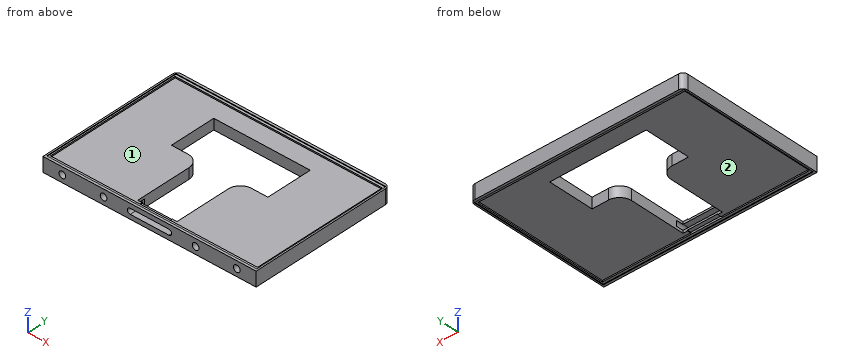
from build123d import *

# Parameters (mm, degrees)
SKETCH_1_W           = 176
SKETCH_1_H           = 120
EXTRUDE_1_DEPTH      = 12
SKETCH_2_W           = 171
SKETCH_2_H           = 112
CUT_EXTRUDE_1_DEPTH  = 1.6
SKETCH_3_W           = 171
SKETCH_3_H           = 112
CUT_EXTRUDE_2_DEPTH  = 1.6
SKETCH_5_W           = 173.4
SKETCH_5_H           = 116
CUT_EXTRUDE_3_DEPTH  = 0.5
SKETCH_6_W           = 173.4
SKETCH_6_H           = 116
CUT_EXTRUDE_4_DEPTH  = 0.5
SKETCH_7_W           = 32.5
SKETCH_7_H           = 56
CUT_EXTRUDE_5_DEPTH  = 108.014765336
SKETCH_8_W           = 25
SKETCH_8_H           = 5
CUT_EXTRUDE_6_DEPTH  = 0.5
SKETCH_9_W           = 25
SKETCH_9_H           = 5
CUT_EXTRUDE_7_DEPTH  = 0.5
FILLET_1_R           = 4
FILLET_2_R           = 4
SKETCH_28_R          = 2.75
CUT_EXTRUDE_16_DEPTH = 5.5
CUT_EXTRUDE_17_DEPTH = 13
SKETCH_31_W          = 79.660251382
SKETCH_31_H          = 38
CUT_EXTRUDE_18_DEPTH = 108.014765336
FILLET_3_R           = 10
FILLET_4_R           = 10


with BuildPart() as part:
    # 草图1 → 凸台-拉伸1 (new body)
    with BuildSketch(Plane.XY):
        Rectangle(SKETCH_1_W, SKETCH_1_H)
    extrude(amount=EXTRUDE_1_DEPTH)

    # 草图2 → 切除-拉伸1 (cut)
    with BuildSketch(Plane.XY.offset(12)):
        Rectangle(SKETCH_2_W, SKETCH_2_H)
    extrude(amount=-CUT_EXTRUDE_1_DEPTH, mode=Mode.SUBTRACT)

    # 草图3 → 切除-拉伸2 (cut)
    with BuildSketch(Plane(origin=(0, 0, 0), x_dir=(-1, 0, 0), z_dir=(0, 0, -1))):
        Rectangle(SKETCH_3_W, SKETCH_3_H)
    extrude(amount=-CUT_EXTRUDE_2_DEPTH, mode=Mode.SUBTRACT)

    # 草图5 → 切除-拉伸3 (cut)
    with BuildSketch(Plane(origin=(0, 0, 0), x_dir=(-1, 0, 0), z_dir=(0, 0, -1))):
        Rectangle(SKETCH_5_W, SKETCH_5_H)
    extrude(amount=-CUT_EXTRUDE_3_DEPTH, mode=Mode.SUBTRACT)

    # 草图6 → 切除-拉伸4 (cut)
    with BuildSketch(Plane.XY.offset(12)):
        Rectangle(SKETCH_6_W, SKETCH_6_H)
    extrude(amount=-CUT_EXTRUDE_4_DEPTH, mode=Mode.SUBTRACT)

    # 草图7 → 切除-拉伸5 (cut, through all)
    with BuildSketch(Plane(origin=(0, 0, 1.6), x_dir=(-1, 0, 0), z_dir=(0, 0, -1))):
        with Locations((0, -25)):
            Rectangle(SKETCH_7_W, SKETCH_7_H)
    extrude(amount=-CUT_EXTRUDE_5_DEPTH, mode=Mode.SUBTRACT)

    # 草图8 → 切除-拉伸6 (cut)
    with BuildSketch(Plane(origin=(0, 0, 1.6), x_dir=(-1, 0, 0), z_dir=(0, 0, -1))):
        with Locations((0, -53.5)):
            Rectangle(SKETCH_8_W, SKETCH_8_H)
    extrude(amount=-CUT_EXTRUDE_6_DEPTH, mode=Mode.SUBTRACT)

    # 草图9 → 切除-拉伸7 (cut)
    with BuildSketch(Plane.XY.offset(10.4)):
        with Locations((0, -53.5)):
            Rectangle(SKETCH_9_W, SKETCH_9_H)
    extrude(amount=-CUT_EXTRUDE_7_DEPTH, mode=Mode.SUBTRACT)

    # 圆角1
    fillet_1_edges = [part.edges().sort_by_distance(p)[0] for p in [
        (-88, 60, 6),
    ]]
    fillet(fillet_1_edges, radius=FILLET_1_R)

    # 圆角2
    fillet_2_edges = [part.edges().sort_by_distance(p)[0] for p in [
        (88, 60, 6),
    ]]
    fillet(fillet_2_edges, radius=FILLET_2_R)

    # 草图28 → 切除-拉伸16 (cut)
    with BuildSketch(Plane(origin=(0, -60, 0), x_dir=(-1, 0, 0), z_dir=(0, -1, 0))):
        with Locations(Location((-72, -6, 0), (0, 0, 180))):
            Circle(SKETCH_28_R)
        with Locations(Location((-38, -6, 0), (0, 0, 180))):
            Circle(SKETCH_28_R)
        with Locations(Location((38, -6, 0), (0, 0, 180))):
            Circle(SKETCH_28_R)
        with Locations(Location((72, -6, 0), (0, 0, 180))):
            Circle(SKETCH_28_R)
    extrude(amount=-CUT_EXTRUDE_16_DEPTH, mode=Mode.SUBTRACT)

    # 草图29 → 切除-拉伸17 (cut)
    with BuildSketch(Plane.XZ.offset(60)):
        with BuildLine():
            Line((-16, 8.25), (16, 8.25))
            ThreePointArc((16, 8.25), (18.25, 6), (16, 3.75))
            Line((16, 3.75), (-16, 3.75))
            ThreePointArc((-16, 3.75), (-18.25, 6), (-16, 8.25))
        make_face()
    extrude(amount=-CUT_EXTRUDE_17_DEPTH, mode=Mode.SUBTRACT)

    # 草图31 → 切除-拉伸18 (cut, through all)
    with BuildSketch(Plane(origin=(0, 0, 1.6), x_dir=(-1, 0, 0), z_dir=(0, 0, -1))):
        with Locations((0, 22)):
            Rectangle(SKETCH_31_W, SKETCH_31_H)
    extrude(amount=-CUT_EXTRUDE_18_DEPTH, mode=Mode.SUBTRACT)

    # 圆角3
    fillet_3_edges = [part.edges().sort_by_distance(p)[0] for p in [
        (-16.25, 3, 6),
    ]]
    fillet(fillet_3_edges, radius=FILLET_3_R)

    # 圆角4
    fillet_4_edges = [part.edges().sort_by_distance(p)[0] for p in [
        (16.25, 3, 6),
    ]]
    fillet(fillet_4_edges, radius=FILLET_4_R)


solid = part.part
Model file for the job. Use its own axes, mm. Face numbers are marked on the shaded views. Coordinates: 2 decimals unless noted, no trailing zeros. Write each loop counter-clockwise with the first axis right and the second up, starting at its lowest first coordinate (ties: lowest second). Pieces come first, ordered by that corner, then holes. Notation, with made-up numbers: (5, 40) -> (49, 40) arc R10 ccw to (49, 48) -> close; hole circle Ø2 at (-40, 12.25). An arc over 180 degrees is marked (long way). One line per item, written item: value. Start each with the question number.
1) Slice it at C-C on y = -20.5. Write the cut outline in (x, z), then the cut area to 3 significant figures.
2) Flat gauge pins, fed straight in: pin 1 Ø0.6 at (x, z) = (17.5, 6) entering from -Y; pin 2 Ø5 at (x, y) = (68.5, 26) entering from -Z; pin 3 Ø0.9 at (x, y) = (-2.5, -55) entering from -Z. Where does each tip first touch, or does it go through?
3) Pull direction X, two halves, no side cores. Call the marked faces 1 and 2: +X half, -X half, draft (parallel to the pull), parting line (faces both ways), or undercut.
4) Slice it at D-D on x = -72. Write the cut outline in (y, z), then the cut area to 3 significant figures.
5) Probe probe 1 along Z at (x, y) = (38, -57.95); probe 2 along X at (y, z) = (35.5, 9.25); probe 3 along X at (y, z) = (-21, 2). List the from-to ranges inside material, lowest first.
6) Slice it at B-B on x = -38. Write the cut outline in (y, z), then the cut area to 3 significant figures.
7) Slice it at A-A on y = 16.5. Write the cut outline in (x, z).
Answers follow:
1. outline: (-88, 0) -> (-86.7, 0) -> (-86.7, 0.5) -> (-85.5, 0.5) -> (-85.5, 1.6) -> (-16.25, 1.6) -> (-16.25, 10.4) -> (-85.5, 10.4) -> (-85.5, 11.5) -> (-86.7, 11.5) -> (-86.7, 12) -> (-88, 12) -> close; (16.25, 1.6) -> (85.5, 1.6) -> (85.5, 0.5) -> (86.7, 0.5) -> (86.7, 0) -> (88, 0) -> (88, 12) -> (86.7, 12) -> (86.7, 11.5) -> (85.5, 11.5) -> (85.5, 10.4) -> (16.25, 10.4) -> close
1. area: 1,280 mm2
2. pin 1: y = -47
2. pin 2: z = 1.6
2. pin 3: z = 2.1
3. face 1: undercut
3. face 2: undercut
4. outline: (-60, 0) -> (-58, 0) -> (-58, 0.5) -> (-56, 0.5) -> (-56, 1.6) -> (56, 1.6) -> (56, 0.5) -> (58, 0.5) -> (58, 0) -> (60, 0) -> (60, 12) -> (58, 12) -> (58, 11.5) -> (56, 11.5) -> (56, 10.4) -> (-56, 10.4) -> (-56, 11.5) -> (-58, 11.5) -> (-58, 12) -> (-60, 12) -> (-60, 8.75) -> (-54.5, 8.75) -> (-54.5, 3.25) -> (-60, 3.25) -> close
4. area: 1,050 mm2
5. probe 1: 0.5 to 3.25, 8.75 to 11.5
5. probe 2: -88 to -39.83, 39.83 to 88
5. probe 3: -88 to -16.25, 16.25 to 88
6. outline: (-60, 0) -> (-58, 0) -> (-58, 0.5) -> (-56, 0.5) -> (-56, 1.6) -> (3, 1.6) -> (3, 10.4) -> (-56, 10.4) -> (-56, 11.5) -> (-58, 11.5) -> (-58, 12) -> (-60, 12) -> (-60, 8.75) -> (-54.5, 8.75) -> (-54.5, 3.25) -> (-60, 3.25) -> close; (41, 1.6) -> (56, 1.6) -> (56, 0.5) -> (58, 0.5) -> (58, 0) -> (60, 0) -> (60, 12) -> (58, 12) -> (58, 11.5) -> (56, 11.5) -> (56, 10.4) -> (41, 10.4) -> close
6. area: 713 mm2
7. outline: (-88, 0) -> (-86.7, 0) -> (-86.7, 0.5) -> (-85.5, 0.5) -> (-85.5, 1.6) -> (-39.83, 1.6) -> (-39.83, 10.4) -> (-85.5, 10.4) -> (-85.5, 11.5) -> (-86.7, 11.5) -> (-86.7, 12) -> (-88, 12) -> close; (39.83, 1.6) -> (85.5, 1.6) -> (85.5, 0.5) -> (86.7, 0.5) -> (86.7, 0) -> (88, 0) -> (88, 12) -> (86.7, 12) -> (86.7, 11.5) -> (85.5, 11.5) -> (85.5, 10.4) -> (39.83, 10.4) -> close
